```python
from build123d import *

# Parameters (mm, degrees)
SKETCH_1_W          = 270
SKETCH_1_H          = 5
EXTRUDE_1_DEPTH     = 95
SKETCH_2_R          = 2.25
SKETCH_2_R_2        = 1.75
SKETCH_2_R_3        = 17.5
SKETCH_2_R_4        = 35
CUT_EXTRUDE_1_DEPTH = 10
SKETCH_3_W          = 70
SKETCH_3_H          = 20
CUT_EXTRUDE_2_DEPTH = 10
FILLET_1_R          = 10
FILLET_2_R          = 20


with BuildPart() as part:
    # 草图1 → 拉伸-薄壁1 (new body)
    with BuildSketch(Plane.XY):
        with Locations((-135, -2.5)):
            Rectangle(SKETCH_1_W, SKETCH_1_H)
    extrude(amount=EXTRUDE_1_DEPTH)

    # 草图2 → 切除-拉伸1 (cut)
    with BuildSketch(Plane(origin=(0, 0, 0), x_dir=(1, 0, 0), z_dir=(0, 1, 0))):
        with Locations(Location((-246, -25.75, 0), (0, 0, 270))):
            Circle(SKETCH_2_R)
        with Locations(Location((-229.338533362, -33.519369489, 0), (0, 0, 270))):
            Circle(SKETCH_2_R)
        with Locations(Location((-262.661466638, -33.519369489, 0), (0, 0, 270))):
            Circle(SKETCH_2_R)
        with Locations(Location((-262.661466638, -61.480630511, 0), (0, 0, 270))):
            Circle(SKETCH_2_R)
        with Locations(Location((-246, -69.25, 0), (0, 0, 270))):
            Circle(SKETCH_2_R)
        with Locations(Location((-229.338533362, -61.480630511, 0), (0, 0, 270))):
            Circle(SKETCH_2_R)
        with Locations(Location((-3.5, -47.5, 0), (0, 0, 270))):
            Circle(SKETCH_2_R_2)
        with Locations(Location((-15.9479618, -77.5520382, 0), (0, 0, 270))):
            Circle(SKETCH_2_R_2)
        with Locations(Location((-46, -90, 0), (0, 0, 270))):
            Circle(SKETCH_2_R_2)
        with Locations(Location((-76.0520382, -77.5520382, 0), (0, 0, 270))):
            Circle(SKETCH_2_R_2)
        with Locations(Location((-88.5, -47.5, 0), (0, 0, 270))):
            Circle(SKETCH_2_R_2)
        with Locations(Location((-76.0520382, -17.4479618, 0), (0, 0, 270))):
            Circle(SKETCH_2_R_2)
        with Locations(Location((-46, -5, 0), (0, 0, 270))):
            Circle(SKETCH_2_R_2)
        with Locations(Location((-15.9479618, -17.4479618, 0), (0, 0, 270))):
            Circle(SKETCH_2_R_2)
        with Locations(Location((-246, -47.5, 0), (0, 0, 270))):
            Circle(SKETCH_2_R_3)
        with Locations(Location((-46, -47.5, 0), (0, 0, 270))):
            Circle(SKETCH_2_R_4)
    extrude(amount=-CUT_EXTRUDE_1_DEPTH, mode=Mode.SUBTRACT)

    # 草图3 → 切除-拉伸2 (cut)
    with BuildSketch(Plane(origin=(0, 0, 0), x_dir=(1, 0, 0), z_dir=(0, 1, 0))):
        with Locations((-235, -85)):
            Rectangle(SKETCH_3_W, SKETCH_3_H)
        with Locations((-235, -10)):
            Rectangle(SKETCH_3_W, SKETCH_3_H)
        with BuildLine():
            Line((-190, -10), (-190, -34.757359313))
            ThreePointArc((-190, -34.757359313), (-188.148050297, -37.52899791), (-184.878679656, -36.878679656))
            Line((-184.878679656, -36.878679656), (-160.121320344, -12.121320344))
            ThreePointArc((-160.121320344, -12.121320344), (-159.47100209, -8.851949703), (-162.242640687, -7))
            Line((-162.242640687, -7), (-187, -7))
            ThreePointArc((-187, -7), (-189.121320344, -7.878679656), (-190, -10))
        make_face()
        with BuildLine():
            Line((-154.121320344, -12.121320344), (-178.878679656, -36.878679656))
            ThreePointArc((-178.878679656, -36.878679656), (-179.52899791, -40.148050297), (-176.757359313, -42))
            Line((-176.757359313, -42), (-152, -42))
            ThreePointArc((-152, -42), (-149.878679656, -41.121320344), (-149, -39))
            Line((-149, -39), (-149, -14.242640687))
            ThreePointArc((-149, -14.242640687), (-150.851949703, -11.47100209), (-154.121320344, -12.121320344))
        make_face()
        with BuildLine():
            Line((-112.242640687, -7), (-137, -7))
            ThreePointArc((-137, -7), (-139.121320344, -7.878679656), (-140, -10))
            Line((-140, -10), (-140, -34.757359313))
            ThreePointArc((-140, -34.757359313), (-138.148050297, -37.52899791), (-134.878679656, -36.878679656))
            Line((-134.878679656, -36.878679656), (-110.121320344, -12.121320344))
            ThreePointArc((-110.121320344, -12.121320344), (-109.47100209, -8.851949703), (-112.242640687, -7))
        make_face()
        with BuildLine():
            Line((-99, -39), (-99, -14.242640687))
            ThreePointArc((-99, -14.242640687), (-100.851949703, -11.47100209), (-104.121320344, -12.121320344))
            Line((-104.121320344, -12.121320344), (-128.878679656, -36.878679656))
            ThreePointArc((-128.878679656, -36.878679656), (-129.52899791, -40.148050297), (-126.757359313, -42))
            Line((-126.757359313, -42), (-102, -42))
            ThreePointArc((-102, -42), (-99.878679656, -41.121320344), (-99, -39))
        make_face()
        with BuildLine():
            Line((-112.242640687, -52), (-137, -52))
            ThreePointArc((-137, -52), (-139.121320344, -52.878679656), (-140, -55))
            Line((-140, -55), (-140, -79.757359313))
            ThreePointArc((-140, -79.757359313), (-138.148050297, -82.52899791), (-134.878679656, -81.878679656))
            Line((-134.878679656, -81.878679656), (-110.121320344, -57.121320344))
            ThreePointArc((-110.121320344, -57.121320344), (-109.47100209, -53.851949703), (-112.242640687, -52))
        make_face()
        with BuildLine():
            Line((-99, -84), (-99, -59.242640687))
            ThreePointArc((-99, -59.242640687), (-100.851949703, -56.47100209), (-104.121320344, -57.121320344))
            Line((-104.121320344, -57.121320344), (-128.878679656, -81.878679656))
            ThreePointArc((-128.878679656, -81.878679656), (-129.52899791, -85.148050297), (-126.757359313, -87))
            Line((-126.757359313, -87), (-102, -87))
            ThreePointArc((-102, -87), (-99.878679656, -86.121320344), (-99, -84))
        make_face()
        with BuildLine():
            Line((-162.242640687, -52), (-187, -52))
            ThreePointArc((-187, -52), (-189.121320344, -52.878679656), (-190, -55))
            Line((-190, -55), (-190, -79.757359313))
            ThreePointArc((-190, -79.757359313), (-188.148050297, -82.52899791), (-184.878679656, -81.878679656))
            Line((-184.878679656, -81.878679656), (-160.121320344, -57.121320344))
            ThreePointArc((-160.121320344, -57.121320344), (-159.47100209, -53.851949703), (-162.242640687, -52))
        make_face()
        with BuildLine():
            Line((-149, -84), (-149, -59.242640687))
            ThreePointArc((-149, -59.242640687), (-150.851949703, -56.47100209), (-154.121320344, -57.121320344))
            Line((-154.121320344, -57.121320344), (-178.878679656, -81.878679656))
            ThreePointArc((-178.878679656, -81.878679656), (-179.52899791, -85.148050297), (-176.757359313, -87))
            Line((-176.757359313, -87), (-152, -87))
            ThreePointArc((-152, -87), (-149.878679656, -86.121320344), (-149, -84))
        make_face()
    extrude(amount=-CUT_EXTRUDE_2_DEPTH, mode=Mode.SUBTRACT)

    # 圆角1
    fillet_1_edges = [part.edges().sort_by_distance(p)[0] for p in [
        (-200, -2.5, 95),
        (-200, -2.5, 0),
        (-200, -2.5, 20),
        (-200, -2.5, 75),
        (-270, -2.5, 75),
        (-270, -2.5, 20),
    ]]
    fillet(fillet_1_edges, radius=FILLET_1_R - 0.0001)  # a hair under: the kernel refuses the full size

    # 圆角2
    fillet_2_edges = [part.edges().sort_by_distance(p)[0] for p in [
        (0, -2.5, 0),
        (0, -2.5, 95),
    ]]
    fillet(fillet_2_edges, radius=FILLET_2_R)


solid = part.part
```
Check sheet for the modelled part. Datum: model origin and axes. Units: mm. A direction names the side the tool comes from. Round coordinates to 2 decimals unless told otherwise and drop trailing zeros. Answer as a JSON object with one key per item and string values.
1. Scan lines: line 1 (X direction, y = -2.6, z = 47.5); line 2 (Z direction, x = -182.5, y = -1.2); line 3 (Z direction, x = -188.5, y = -2.05). Record each from-to range of solid material in increasing order.
Reply:
{"line 1": "x = -270 to -263.5, -228.5 to -90.25, -86.75 to -81, -11 to -5.25, -1.75 to 0", "line 2": "z = 0 to 7, 34.5 to 52, 79.5 to 95", "line 3": "z = 0 to 7.4, 37.36 to 52.4, 82.36 to 95"}
2. Section check A-A (y = -1.6). State how many separate pieces and enclosed holes the cut face has, plus the area to 3 significant figures.
Reply:
{"separate pieces": "1", "enclosed holes": "24", "area": "12,900 mm²"}
3. Mould release check, pull along X, two halves, no side actions. Record for faces 3 (the flat face through (-173, -2, 70)), 4 (the cylindrical face through (-203.01, -2.54, 17.15)), 5 (the cylindrical face through (-5.703, -2.465, 88.986)), 6 (the flat face through (-137, -5, 47)): pulls with the +X half, pulls with the -X half, needs draft (parallel to the pull), parting line crosses it, or undercut.
Reply:
{"face 3": "undercut", "face 4": "pulls with the -X half", "face 5": "pulls with the +X half", "face 6": "needs draft"}
4. Access from +Z, -Z, +X, -X, +Y, -Y to the whole of each face (thin tool, end or side, straight path). Record for faces 1 (the flat face through (-137, 0, 47)), 2 (the cylindrical face through (-138.19, -2.46, 82.51)).
Reply:
{"face 1": "+Z, -Z, +X, -X, +Y", "face 2": "+Y, -Y"}
